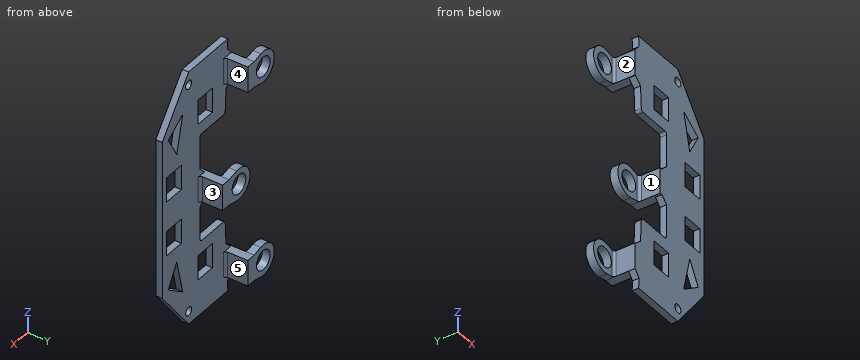
```python
from build123d import *

# Parameters (mm, degrees)
RESSALTO_EXTRUS_O1_DEPTH = 1.25
ESBO_O8_R                = 1.65
ESBO_O8_W                = 8
ESBO_O8_H                = 9.5
CORTE_EXTRUS_O6_DEPTH    = 56.876112964
CORTE_EXTRUS_O5_DEPTH    = 10
RESSALTO_EXTRUS_O4_START = -1.25
ESBO_O12_W               = 3.5
ESBO_O12_H               = 10
RESSALTO_EXTRUS_O4_DEPTH = 11.25
ESBO_O13_R               = 3.75
RESSALTO_EXTRUS_O5_DEPTH = 3
RESSALTO_EXTRUS_O6_START = -11.25
ESBO_O14_W               = 3.5
ESBO_O14_H               = 10
RESSALTO_EXTRUS_O6_DEPTH = 11.25
ESBO_O15_R               = 3.75
RESSALTO_EXTRUS_O7_DEPTH = 3
CHANFRO1_SIZE            = 2.5
CHANFRO1_SIZE_2          = 2.378287199
CHANFRO1_SIZE_3          = 2.642541332
FILETE1_R                = 1


with BuildPart() as part:
    # Esboço1 → Ressalto-extrusão1 (new, symmetric)
    with BuildSketch(Plane(origin=(0, 0, 0), x_dir=(1, 0, 0), z_dir=(0, 1, 0))):
        Polygon((-10.5, -21), (-10.5, 21), (-24.3, 21), (-25.8, 49.5), (-4.3, 49.5), (10.2, 30.65), (10.2, -30.65), (-4.3, -49.5), (-25.8, -49.5), (-24.3, -21), align=None)
    extrude(amount=RESSALTO_EXTRUS_O1_DEPTH, both=True)

    # Esboço8 → Corte-extrusão6 (cut, through all)
    with BuildSketch(Plane(origin=(0, 1.25, 0), x_dir=(1, 0, 0), z_dir=(0, 1, 0))):
        with Locations(Location((-4.3, 44.5, 0), (0, 0, 270))):
            Circle(ESBO_O8_R)
        with Locations((-13.3, 30.55)):
            Rectangle(ESBO_O8_W, ESBO_O8_H)
        with Locations((3.75, 10.55)):
            Rectangle(ESBO_O8_W, ESBO_O8_H)
    corte_extrus_o6 = extrude(amount=-CORTE_EXTRUS_O6_DEPTH, mode=Mode.SUBTRACT)

    # Esboço9 → Corte-extrusão5 (cut)
    with BuildSketch(Plane(origin=(0, 1.25, 0), x_dir=(1, 0, 0), z_dir=(0, 1, 0))):
        Polygon((6.901537023, 29.384909169), (-1.046130524, 34.9078029), (2.24312, 21.07143213), align=None)
    corte_extrus_o5 = extrude(amount=-CORTE_EXTRUS_O5_DEPTH, mode=Mode.SUBTRACT)

    # Esboço12 → Ressalto-extrusão4 (add)
    with BuildSketch(Plane(origin=(0, 0, 0), x_dir=(1, 0, 0), z_dir=(0, 1, 0)).offset(RESSALTO_EXTRUS_O4_START)):
        with Locations((-26.05, 38)):
            Rectangle(ESBO_O12_W, ESBO_O12_H)
    ressalto_extrus_o4 = extrude(amount=RESSALTO_EXTRUS_O4_DEPTH)

    # Esboço13 → Ressalto-extrusão5 (add)
    with BuildSketch(Plane(origin=(0, 10, 0), x_dir=(1, 0, 0), z_dir=(0, 1, 0))):
        with BuildLine():
            Line((-31.444994432, 43.844994432), (-27.8, 43))
            Line((-27.8, 43), (-27.8, 33))
            Line((-27.8, 33), (-31.444994432, 32.155005568))
            ThreePointArc((-31.444994432, 32.155005568), (-38.8, 38), (-31.444994432, 43.844994432))
        make_face()
        with Locations(Location((-32.8, 38, 0), (0, 0, 270))):
            Circle(ESBO_O13_R, mode=Mode.SUBTRACT)
    ressalto_extrus_o5 = extrude(amount=-RESSALTO_EXTRUS_O5_DEPTH)

    # Espelhar1: Corte-extrusão6, Corte-extrusão5, Ressalto-extrusão4, Ressalto-extrusão5 across plane
    add(corte_extrus_o6.mirror(Plane.XY), mode=Mode.SUBTRACT)
    add(corte_extrus_o5.mirror(Plane.XY), mode=Mode.SUBTRACT)
    add(ressalto_extrus_o4.mirror(Plane.XY))
    add(ressalto_extrus_o5.mirror(Plane.XY))

    # Esboço14 → Ressalto-extrusão6 (add)
    with BuildSketch(Plane.XZ.offset(1.25).offset(RESSALTO_EXTRUS_O6_START)):
        with Locations((-12.25, 0)):
            Rectangle(ESBO_O14_W, ESBO_O14_H)
    extrude(amount=RESSALTO_EXTRUS_O6_DEPTH)

    # Esboço15 → Ressalto-extrusão7 (add)
    with BuildSketch(Plane(origin=(0, 10, 0), x_dir=(1, 0, 0), z_dir=(0, 1, 0))):
        with BuildLine():
            Line((-18.247793537, 5.876270543), (-14, 5))
            Line((-14, 5), (-14, -5))
            Line((-14, -5), (-18.247793537, -5.876270543))
            ThreePointArc((-18.247793537, -5.876270543), (-25.46, 0), (-18.247793537, 5.876270543))
        make_face()
        with Locations(Location((-19.46, 0, 0), (0, 0, 270))):
            Circle(ESBO_O15_R, mode=Mode.SUBTRACT)
    extrude(amount=-RESSALTO_EXTRUS_O7_DEPTH)

    # Chanfro1
    # the kernel refuses this chamfer: 2.642541332, 2.5, 2.378287199 mm, written as the material it adds along each edge
    with BuildSketch(Plane(origin=(-10.5, 1.25, -5), x_dir=(0.02749587661058631, 0, -0.9996219169112968), z_dir=(0, -1, 0))) as chanfro1_piece_1:
        Polygon((CHANFRO1_SIZE * 0.999621916911, -CHANFRO1_SIZE * 0.0274958766106), (-CHANFRO1_SIZE * 0.0274958766106, -CHANFRO1_SIZE * 0.999621916911), (0, 0), align=None)
    extrude(amount=2.5)
    with BuildSketch(Plane(origin=(-10.5, 1.25, 5), x_dir=(0.02749587661058631, 0, 0.9996219169112968), z_dir=(0, -1, 0))) as chanfro1_piece_2:
        Polygon((CHANFRO1_SIZE * 0.999621916911, CHANFRO1_SIZE * 0.0274958766106), (-CHANFRO1_SIZE * 0.0274958766106, CHANFRO1_SIZE * 0.999621916911), (0, 0), align=None)
    extrude(amount=2.5)
    with BuildSketch(Plane(origin=(-25.457894737, 1.25, 43), x_dir=(-0.9995382917887814, 0, -0.03038425987192659), z_dir=(0, -1, 0))) as chanfro1_piece_3_section:
        Polygon((CHANFRO1_SIZE_2 * 0.999538291707, -CHANFRO1_SIZE_2 * 0.0303842598694), (CHANFRO1_SIZE * 0.0221923026388, -CHANFRO1_SIZE * 0.999753720525), (0, 0), align=None)
    chanfro1_piece_3 = extrude(amount=2.5, mode=Mode.PRIVATE)
    chanfro1_piece_3 = split(chanfro1_piece_3, bisect_by=Plane(origin=(-27.8, 0, 43.832382162), z_dir=(1, 0, 0)), keep=Keep.TOP, mode=Mode.PRIVATE)
    add(chanfro1_piece_3)
    with BuildSketch(Plane(origin=(-24.931578947, -1.25, 33), x_dir=(0.0815134342344048, 0, -0.9966722430364525), z_dir=(0, 1, 0))) as chanfro1_piece_4:
        Polygon((CHANFRO1_SIZE * 0.999578922884, CHANFRO1_SIZE * 0.0290168386568), (-CHANFRO1_SIZE_3 * 0.0815134342346, CHANFRO1_SIZE_3 * 0.996672243039), (0, 0), align=None)
    extrude(amount=2.5)
    with BuildSketch(Plane(origin=(-25.457894737, 1.25, -43), x_dir=(-0.025081088900339724, 0, -0.9996854200095016), z_dir=(0, -1, 0))) as chanfro1_piece_5_section:
        Polygon((CHANFRO1_SIZE * 0.999621916911, -CHANFRO1_SIZE * 0.0274958766106), (CHANFRO1_SIZE_2 * 0.0250810888983, -CHANFRO1_SIZE_2 * 0.999685419928), (0, 0), align=None)
    chanfro1_piece_5 = extrude(amount=2.5, mode=Mode.PRIVATE)
    chanfro1_piece_5 = split(chanfro1_piece_5, bisect_by=Plane(origin=(-27.8, 0, -43.832382162), z_dir=(1, 0, 0)), keep=Keep.TOP, mode=Mode.PRIVATE)
    add(chanfro1_piece_5)
    with BuildSketch(Plane(origin=(-24.931578947, -1.25, -33), x_dir=(-0.9996625353173835, 0, -0.0259772108360549), z_dir=(0, 1, 0))) as chanfro1_piece_6:
        Polygon((CHANFRO1_SIZE_3 * 0.99966253532, CHANFRO1_SIZE_3 * 0.0259772108361), (-CHANFRO1_SIZE * 0.07848240227, CHANFRO1_SIZE * 0.996915499194), (0, 0), align=None)
    extrude(amount=2.5)

    # Filete1
    filete1_edges = [part.edges().sort_by_distance(p)[0] for p in [
        (-27.8, 7, -38),
        (-14, 7, 0),
        (-27.8, 7, 38),
        (-24.3, 1.25, -38),
        (-10.5, 1.25, 0),
        (-24.3, 1.25, 38),
        (-24.3, 0, 21),
        (-10.5, 0, 21),
        (-10.5, 0, -21),
        (-24.3, 0, -21),
    ]]
    fillet(filete1_edges, radius=FILETE1_R)


solid = part.part
```
Can you work these out from the model? Positions are in its coordinate system, mm. Face numbers are marked on the shaded views. A direction names the side the tool comes from. Round coordinates to 2 decimals unless told otherwise and drop trailing zeros. Loops run counter-clockwise (first coordinate to the right, second up) from the corner with the lowest first, then second, coordinate; pieces in that order, holes last. Notation, with made-up numbers: M 31,36 L 80,36 A32 ccw 80,74 Z; hole C 35,-18.5 d10. An arc over 180 degrees is marked long. Answer in a Markdown table with one row per item.
1. I'm going to push flat-ended pins straight in: pin 1 Ø4.5 at (x, z) = (-4.3, -44.5) entering from +Y; pin 2 Ø1 at (y, z) = (4, 6.5) entering from +X; pin 3 Ø2 at (x, y) = (3, -0.5) entering from +Z; pin 4 Ø0.8 at (y, z) = (0, 33) entering from -X. Where does each tip first touch, or does it pass through?
Established:
| item | result |
|---|---|
| pin 1 | y = 1.25 |
| pin 2 | through |
| pin 3 | z = 41.31 |
| pin 4 | x = -27.8 |
2. Please list where these lines run through material, in increasing order: line 1 (X direction, y = 9.3, z = -38); line 2 (Z direction, x = -5, y = 0.25); line 3 (Z direction, x = 4, y = 0). Write a range as from..to.
Established:
| item | result |
|---|---|
| line 1 | -38.8..-36.55, -29.05..-24.3 |
| line 2 | -49.5..-45.99, -43.01..43.01, 45.99..49.5 |
| line 3 | -38.71..-31.4, -24.21..-15.3, -5.8..5.8, 15.3..24.21, 31.4..38.71 |
3. If we section it at B-B, the plane z = 0: Please give me the cut outline in (x, y).
Established:
| item | result |
|---|---|
| outline | M -25.46,7 L -23.21,7 L -23.21,10 L -25.46,10 Z; M -15.71,7 L -15,7 A1 cw -14,6 L -14,-1.25 L 10.2,-1.25 L 10.2,1.25 L -9.5,1.25 A1 cw -10.5,2.25 L -10.5,10 L -15.71,10 Z |
4. If we section it at C-C, the plane x = -32.8: Please give me the cut outline in (y, z).
Established:
| item | result |
|---|---|
| outline | M 7,-44 L 10,-44 L 10,-41.75 L 7,-41.75 Z; M 7,-34.25 L 10,-34.25 L 10,-32 L 7,-32 Z; M 7,32 L 10,32 L 10,34.25 L 7,34.25 Z; M 7,41.75 L 10,41.75 L 10,44 L 7,44 Z |
5. On a 3-axis mill with a long thin cutter (end or side, diameter ignored), from which of +Z, -Z, +X, -X, +Y, -Y can I reach the whole of each face in a straight line? I mean the marked faces 1, 2, 3, 4 and 5. Say none if no direction works.
Established:
| item | result |
|---|---|
| face 1 | -X, -Y |
| face 2 | +Z, -Z, -X, -Y |
| face 3 | +Z, -Z, +X, +Y |
| face 4 | +Z, +X, +Y |
| face 5 | -Z, +X, +Y |
6. If we section it at D-D, the plane y = 5: Please give me the cut outline in (x, z).
Established:
| item | result |
|---|---|
| outline | M -27.8,-43 L -24.3,-43 L -24.3,-33 L -27.8,-33 Z; M -27.8,33 L -24.3,33 L -24.3,43 L -27.8,43 Z; M -14,-5 L -10.5,-5 L -10.5,5 L -14,5 Z |
7. If we section it at A-A, the plane y = 9: Please give me the cut outline in (x, z) (3 decimals), plus the area to 3 significant figures.
Established:
| item | result |
|---|---|
| outline | M -31.445,-43.845 L -27.8,-43 L -24.3,-43 L -24.3,-33 L -27.8,-33 L -31.445,-32.155 A6 ccw long Z; M -31.445,32.155 L -27.8,33 L -24.3,33 L -24.3,43 L -27.8,43 L -31.445,43.845 A6 ccw long Z; M -18.248,-5.876 L -14,-5 L -10.5,-5 L -10.5,5 L -14,5 L -18.248,5.876 A6 ccw long Z; hole C -32.8,-38 d7.5; hole C -32.8,38 d7.5; hole C -19.46,0 d7.5 |
| area | 314 mm² |
